Can you work these out from the model? Positions are in its coordinate system, mm. A direction names the side the tool comes from. Give positions to 0.01 mm unless a question says otherwise; leave off trailing zeros. Write each loop counter-clockwise with the first axis right and the second up, starting at its lowest first coordinate (ties: lowest second). Pieces come first, ordered by that corner, then holes. Notation, with made-up numbers: M -4.5,86.5 L 54.5,86.5 A27 cw 54.5,115.5 Z; hole C -23,11 d5. An arc over 180 degrees is marked long. Write each question's results on one line, items separated by ' | '.
from build123d import *

# Parameters (mm, degrees)
SKETCH2_R               = 1
BOSS_EXTRUDE2_DEPTH     = 30
CUT_EXTRUDE1_DEPTH      = 37.224991373
CUT_EXTRUDE1_DEPTH_BACK = 37.224991373
SKETCH3_R               = 2.15
SKETCH3_W               = 10
SKETCH3_H               = 7


with BuildPart() as part:
    # Sketch2 → Boss-Extrude2 (new body)
    with BuildSketch(Plane.XY):
        with BuildLine():
            Line((1, 3.5), (1, 20))
            Line((1, 20), (2.5, 20))
            Line((2.5, 20), (2.5, 0))
            ThreePointArc((2.5, 0), (-1.767766953, -1.767766953), (0, 2.5))
            ThreePointArc((0, 2.5), (0.707106781, 2.792893219), (1, 3.5))
        make_face()
        Circle(SKETCH2_R, mode=Mode.SUBTRACT)
    extrude(amount=BOSS_EXTRUDE2_DEPTH)

    # Sketch3 → Cut-Extrude1 (cut, two sides: drawn at the far end of the back side and taken through both)
    with BuildSketch(Plane.ZY.offset(-1).offset(-CUT_EXTRUDE1_DEPTH_BACK)):
        with Locations(Location((7.5, 15.5, 0), (0, 0, 270))):
            Circle(SKETCH3_R)
        with Locations(Location((22.5, 15.5, 0), (0, 0, 270))):
            Circle(SKETCH3_R)
        with Locations((5, 0)):
            Rectangle(SKETCH3_W, SKETCH3_H)
        with Locations((25, 0)):
            Rectangle(SKETCH3_W, SKETCH3_H)
    extrude(amount=CUT_EXTRUDE1_DEPTH + CUT_EXTRUDE1_DEPTH_BACK, mode=Mode.SUBTRACT)


solid = part.part
Item 1: For faces 1 (the face through (1, 12, 15)), 2 (the face through (2, 12, 0)), 3 (the face through (2, 3.5, 5)), which set-ups out of +Z, -Z, +X, -X, +Y, -Y let a thin tool reach every point of the face, with its end or its side?
Geometry says:
face 1: +Z, -Z, -X, +Y | face 2: -Z, +X, -X, +Y, -Y | face 3: -Z, +X, -X, -Y
Item 2: I want a section at D-D, the plane z = 13.25. Please give me the cut outline in (x, y), and give its area (3 significant figures).
Geometry says:
outline: M 0,2.5 A2.5 ccw long 2.5,0 L 2.5,20 L 1,20 L 1,3.5 A1 cw Z; hole C 0,0 d2 | area: 44.3 mm2
Item 3: If I drill on line 1 (Y direction, x = 2, z = 22.5); line 2 (Z direction, x = 1.5, y = 15.5); line 3 (X direction, y = 0, z = 14), over which ranges is the centre line in solid material (lowest first)? Write a range as from..to.
Geometry says:
line 1: y = 3.5..13.35, 17.65..20 | line 2: z = 0..5.35, 9.65..20.35, 24.65..30 | line 3: x = -2.5..-1, 1..2.5
Item 4: I want a section at B-B, the plane z = 22.5. Please give me the cut outline in (x, y), and give its area (3 significant figures).
Geometry says:
outline: M 1,3.5 L 2.5,3.5 L 2.5,13.35 L 1,13.35 Z; M 1,17.65 L 2.5,17.65 L 2.5,20 L 1,20 Z | area: 18.3 mm2
Item 5: I want a section at C-C, the plane x = 1.5. Please give me the cut outline in (y, z).
Geometry says:
outline: M -2,10 L 3.5,10 L 3.5,0 L 20,0 L 20,30 L 3.5,30 L 3.5,20 L -2,20 Z; hole C 15.5,7.5 d4.3; hole C 15.5,22.5 d4.3
Item 6: Thinking about a two-plate mould opening in Y: for faces 4 (the face through (1, 1, 20)), 5 (the face through (2, 3.5, 25)), 6 (the face through (1.76, 14.34, 9.31)), which applies, +Y half, -Y half, draft (parallel to the pull), parting line (faces both ways), or undercut?
Geometry says:
face 4: draft | face 5: -Y half | face 6: undercut
Item 7: I'm going to push flat-ended pins straight in: pin 1 (1.5 mm diameter, centred on x = 1, y = 1.5, fed in from -Z); pin 2 (7 mm diameter, centred on y = 15.5, z = 7.5, fed in from -X); pin 3 (1.8 mm diameter, centred on x = 0, y = 0, fed in from +Z); pin 4 (0.8 mm diameter, centred on x = 2, z = 4, fed in from -Y). Where does each tip first touch, or does it pass through?
Geometry says:
pin 1: stops at z = 10 | pin 2: stops at x = 1 | pin 3: passes through | pin 4: stops at y = 3.5
Item 8: I want a section at A-A, the plane y = 15.5. Please give me the cut outline in (x, z).
Geometry says:
outline: M 1,0 L 2.5,0 L 2.5,5.35 L 1,5.35 Z; M 1,9.65 L 2.5,9.65 L 2.5,20.35 L 1,20.35 Z; M 1,24.65 L 2.5,24.65 L 2.5,30 L 1,30 Z
